Can you work these out from the model? Positions are in its coordinate system, mm. Face numbers are marked on the shaded views. Coordinates: 2 decimals unless noted, no trailing zeros. Order: outer loops, then holes, each group sorted by start corner. A loop starts at its lowest first (then second) coordinate and runs counter-clockwise, first axis right, second up. Notation, with made-up numbers: (-31.5, -6) - (15.5, -6) arc R9 cw to (15.5, 9) - close; hole circle Ø1 at (-20.5, -35.75). An arc over 180 degrees is marked (long way). Return JSON: item names as keys, results as strings. Group by question number.
1) If I drill on line 1 along X through (y, z) = (16.5, -6.5); line 2 along Y through (x, z) = (56, -4.5); line 3 along Z through (x, y) = (50, 25.5), over which ranges is the centre line in solid material (lowest first)?
2) Imagine slicing it at C-C (z = -19). Write out the boundary of the cut face in (x, y), and give its area (3 significant figures).
3) If we mould it in two halves opening along X, with no side actions, what happens to the marked faces 1 and 2? For each: pulls with the +X half, pulls with the -X half, needs draft (parallel to the pull), parting line crosses it, or undercut.
4) Imagine slicing it at A-A (x = -26.5). Write out the boundary of the cut face in (y, z).
5) Imagine slicing it at B-B (y = 10). Write out the boundary of the cut face in (x, z), and give its area (3 significant figures).
6) For pin 1 Ø12 at (x, z) = (-9.5, -25.5) entering from -Y; pin 2 Ø8.5 at (y, z) = (10, -13) entering from +X; pin 3 Ø1.5 at (x, z) = (25, -8.5) entering from +Y, each with a flat end and sliding along its axis, tell me the tip position at first contact or that it passes through.
```python
from build123d import *

# Parameters (mm, degrees)
SKETCH018_W             = 120
SKETCH018_H             = 45
PAD003_DEPTH            = 3
SKETCH019_W             = 113.5
SKETCH019_H             = 40
PAD004_DEPTH            = 6
SKETCH020_R             = 1.4
POCKET008_DEPTH         = 116.751
POCKET012_DEPTH         = 376.952357
CHAMFER008_SIZE         = 2
SKETCH021_W             = 105
SKETCH021_H             = 37
POCKET013_DEPTH         = 6
CHAMFER009_SIZE         = 2
CHAMFER010_SIZE         = 1
CHAMFER011_SIZE         = 1
CHAMFER012_SIZE         = 2
BODY001_PLACEMENT_ANGLE = 50


with BuildPart() as part:
    # Sketch018 → Pad003 (new body)
    with BuildSketch(Plane.XZ):
        Rectangle(SKETCH018_W, SKETCH018_H)
    extrude(amount=PAD003_DEPTH)

    # Sketch019 (on Face6 of Pad003) → Pad004 (join)
    with BuildSketch(Plane.XZ.offset(3)):
        Rectangle(SKETCH019_W, SKETCH019_H)
    extrude(amount=PAD004_DEPTH)

    # Sketch020 (on Face8 of Pad004) → Pocket008 (cut, through all)
    with BuildSketch(Plane(origin=(56.75, 0, 0), x_dir=(0, 0, 1), z_dir=(1, 0, 0))):
        with Locations((0, 6)):
            Circle(SKETCH020_R)
    extrude(amount=-POCKET008_DEPTH, mode=Mode.SUBTRACT)

    # Sketch024 (on Face3 of Pocket008) → Pocket012 (cut, through all)
    with BuildSketch(Plane(origin=(60, 0, 0), x_dir=(0, 0, 1), z_dir=(1, 0, 0))):
        Polygon((-22.5, 3), (-17.875456, -3.604533), (-35.516254, -3.604533), align=None)
    pocket012 = extrude(amount=-POCKET012_DEPTH, mode=Mode.SUBTRACT)

    # Mirrored: Pocket012 across Sketch024 V_Axis
    add(pocket012.mirror(Plane(origin=(60, 0, 0), x_dir=(1, 0, 0), z_dir=(0, 0, 1))), mode=Mode.SUBTRACT)

    # Chamfer008
    chamfer008_edges = [part.edges().sort_by_distance(p)[0] for p in [
        (60, 0, 0),
        (-60, 0, 0),
    ]]
    chamfer(chamfer008_edges, length=CHAMFER008_SIZE)

    # Sketch021 → Pocket013 (cut)
    with BuildSketch(Plane.XZ.offset(9)):
        Rectangle(SKETCH021_W, SKETCH021_H)
    extrude(amount=-POCKET013_DEPTH, mode=Mode.SUBTRACT)

    # Chamfer009
    chamfer009_edges = [part.edges().sort_by_distance(p)[0] for p in [
        (-56.75, -6, -20),
    ]]
    chamfer(chamfer009_edges, length=CHAMFER009_SIZE)

    # Chamfer010
    chamfer010_edges = [part.edges().sort_by_distance(p)[0] for p in [
        (56.75, -6, -20),
    ]]
    chamfer(chamfer010_edges, length=CHAMFER010_SIZE)

    # Chamfer011
    chamfer011_edges = [part.edges().sort_by_distance(p)[0] for p in [
        (56.75, -6, 20),
    ]]
    chamfer(chamfer011_edges, length=CHAMFER011_SIZE)

    # Chamfer012
    chamfer012_edges = [part.edges().sort_by_distance(p)[0] for p in [
        (-56.75, -6, 20),
    ]]
    chamfer(chamfer012_edges, length=CHAMFER012_SIZE)


with BuildPart() as part_1:
    # Body001 placement: moved
    add(part.part.moved(Location((7, 16.629636, -17.350208))).rotate(Axis((7, 16.629636, -17.350208), (-1, 0, 0)), BODY001_PLACEMENT_ANGLE))


solid = part_1.part
```
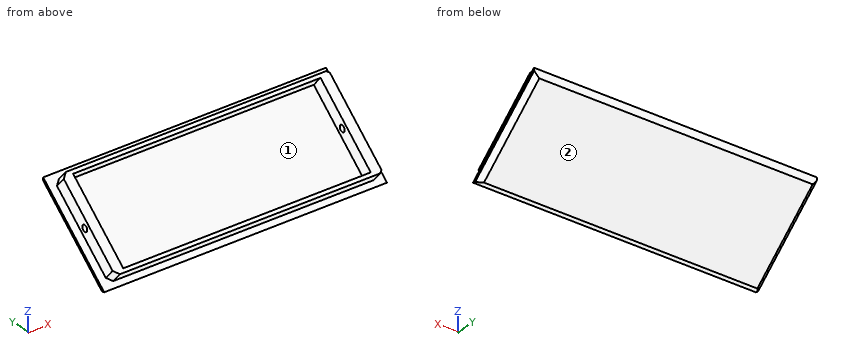
Calculated:
{
 "1": {"line 1": "-49.75 to -45.5, 59.5 to 63.75", "line 2": "27.28 to 31.94", "line 3": "-9.91 to -5.99, 0.86 to 1.84"},
 "2": {"outline": "(-53, 10) - (-49.75, 10) - (-49.75, 0.66) - (-45.5, 0.66) - (-45.5, 10) - (59.5, 10) - (59.5, 0.66) - (63.75, 0.66) - (63.75, 10) - (67, 10) - (67, 11.55) - (65, 14.66) - (-51, 14.66) - (-53, 11.55) - close", "area": "633 mm2"},
 "3": {"face 1": "undercut", "face 2": "needs draft"},
 "4": {"outline": "(-4.48, -23.31) - (-0.62, -27.91) - (-2.53, -29.51) - (1, -30.46) - (32.26, -4.24) - (31.94, -0.59) - (30.02, -2.2) - (26.17, 2.4) - (25.02, 1.44) - (28.87, -3.16) - (0.53, -26.94) - (-3.33, -22.35) - close"},
 "5": {"outline": "(-53, -20.3) - (-51, -22.91) - (65, -22.91) - (67, -20.3) - (67, -19) - (63.75, -19) - (63.75, -11.16) - (59.5, -11.16) - (59.5, -19) - (-45.5, -19) - (-45.5, -11.16) - (-49.75, -11.16) - (-49.75, -19) - (-53, -19) - close", "area": "531 mm2"},
 "6": {"pin 1": "y = -4.48", "pin 2": "x = 63.75", "pin 3": "y = 28.07"}
}
